Autodesk Inventor part; units mm, degrees
ref_plane "YZ Plane" through (0, 0, 0) normal (1, 0, 0) x (0, 1, 0)
ref_plane "XZ Plane" through (0, 0, 0) normal (0, 1, 0) x (-1, 0, 0)
ref_plane "XY Plane" through (0, 0, 0) normal (0, 0, 1) x (1, 0, 0)
sketch "Sketch1" plane through (0, 0, 0) normal (0, 1, 0) x (-1, 0, 0)
  circle A0 centre (225.7737, 188.8152) radius 1.5
  circle A1 centre (325.7737, 262.422) radius 1.5
  circle A2 centre (374.8449, 262.422) radius 1.5
  circle A3 centre (374.8449, 188.8152) radius 1.5
  circle A4 centre (274.8449, 38.8152) radius 1.5
  circle A5 centre (225.7737, 38.8152) radius 1.5
  circle A6 centre (225.7737, 112.422) radius 1.5
  circle A7 centre (325.7737, 38.8152) radius 1.5
  circle A8 centre (374.8449, 38.8152) radius 1.5
  circle A9 centre (374.8449, 112.422) radius 1.5
  line L0 (200.3093, 45.6186) -> (211.8093, 45.6186)
  line L1 (211.8093, 45.6186) -> (223.3093, 45.6186)
  line L2 (377.3093, 45.6186) -> (388.8093, 45.6186)
  line L3 (388.8093, 45.6186) -> (400.3093, 45.6186)
  line L4 (200.3093, 195.6186) -> (211.8093, 195.6186)
  line L5 (211.8093, 195.6186) -> (223.3093, 195.6186)
  line L6 (377.3093, 195.6186) -> (388.8093, 195.6186)
  line L7 (388.8093, 195.6186) -> (400.3093, 195.6186)
  line L8 (294.3093, 194.1186) -> (306.3093, 194.1186)
  line L9 (306.3093, 194.1186) -> (306.3093, 220.1186)
  line L10 (306.3093, 220.1186) -> (294.3093, 220.1186)
  line L11 (294.3093, 220.1186) -> (294.3093, 194.1186)
  arc A10 (278.5735, 87.7325) -> (322.2559, 87.7325) centre (300.4147, 87.7325) ccw
  circle A11 centre (300.4147, 262.422) radius 10
  line L12 (322.2559, 87.7325) -> (322.2559, 139.8246)
  line L13 (322.2559, 139.8246) -> (278.5735, 139.8246)
  line L14 (278.5735, 139.8246) -> (278.5735, 87.7325)
  circle A12 centre (274.8449, 262.422) radius 1.5
  circle A13 centre (225.7737, 262.422) radius 1.5
  line L15 (238.3093, 105.6186) -> (238.3093, 94.1186)
  line L16 (235.3093, 82.6186) -> (238.3093, 82.6186)
  line L17 (238.3093, 82.6186) -> (238.3093, 94.1186)
  line L18 (362.3093, 105.6186) -> (362.3093, 94.1186)
  line L19 (365.3093, 82.6186) -> (362.3093, 82.6186)
  line L20 (362.3093, 82.6186) -> (362.3093, 94.1186)
  line L21 (235.3093, 195.6186) -> (238.3093, 195.6186)
  line L22 (238.3093, 195.6186) -> (238.3093, 207.1186)
  line L23 (235.3093, 218.6186) -> (238.3093, 218.6186)
  line L24 (238.3093, 218.6186) -> (238.3093, 207.1186)
  line L25 (365.3093, 195.6186) -> (362.3093, 195.6186)
  line L26 (362.3093, 195.6186) -> (362.3093, 207.1186)
  line L27 (365.3093, 218.6186) -> (362.3093, 218.6186)
  line L28 (362.3093, 218.6186) -> (362.3093, 207.1186)
  line L29 (365.3093, 105.6186) -> (362.3093, 105.6186)
  arc A14 (300.3093, 0.6186) -> (400.3093, 38.8152) centre (300.3093, 150.6186) ccw
  arc A15 (200.3093, 38.8152) -> (300.3093, 0.6186) centre (300.3093, 150.6186) ccw
  line L30 (235.3093, 105.6186) -> (200.3093, 105.6186)
  line L31 (200.3093, 45.6186) -> (235.3093, 45.6186)
  line L32 (235.3093, 45.6186) -> (235.3093, 82.6186)
  arc A16 (300.3093, 300.6186) -> (200.3093, 262.422) centre (300.3093, 150.6186) ccw
  line L33 (235.3093, 195.6186) -> (200.3093, 195.6186)
  line L34 (200.3093, 255.6186) -> (235.3093, 255.6186)
  line L35 (235.3093, 255.6186) -> (235.3093, 218.6186)
  line L36 (365.3093, 105.6186) -> (400.3093, 105.6186)
  line L37 (400.3093, 45.6186) -> (365.3093, 45.6186)
  line L38 (365.3093, 45.6186) -> (365.3093, 82.6186)
  arc A17 (400.3093, 262.422) -> (300.3093, 300.6186) centre (300.3093, 150.6186) ccw
  line L39 (365.3093, 195.6186) -> (400.3093, 195.6186)
  line L40 (400.3093, 255.6186) -> (365.3093, 255.6186)
  line L41 (365.3093, 255.6186) -> (365.3093, 218.6186)
  line L42 (235.3093, 105.6186) -> (238.3093, 105.6186)
  line L43 (339.9093, 94.1186) -> (339.9093, 105.6186)
  line L44 (339.9093, 105.6186) -> (342.9093, 105.6186)
  line L45 (342.9093, 105.6186) -> (342.9093, 94.1186)
  line L46 (339.9093, 94.1186) -> (339.9093, 82.6186)
  line L47 (339.9093, 82.6186) -> (342.9093, 82.6186)
  line L48 (342.9093, 82.6186) -> (342.9093, 94.1186)
  line L49 (339.9093, 207.1186) -> (339.9093, 195.6186)
  line L50 (339.9093, 195.6186) -> (342.9093, 195.6186)
  line L51 (342.9093, 195.6186) -> (342.9093, 207.1186)
  line L52 (339.9093, 207.1186) -> (339.9093, 218.6186)
  line L53 (339.9093, 218.6186) -> (342.9093, 218.6186)
  line L54 (342.9093, 218.6186) -> (342.9093, 207.1186)
  line L55 (260.7093, 94.1186) -> (260.7093, 105.6186)
  line L56 (260.7093, 105.6186) -> (257.7093, 105.6186)
  line L57 (257.7093, 105.6186) -> (257.7093, 94.1186)
  line L58 (260.7093, 94.1186) -> (260.7093, 82.6186)
  line L59 (260.7093, 82.6186) -> (257.7093, 82.6186)
  line L60 (257.7093, 82.6186) -> (257.7093, 94.1186)
  line L61 (260.7093, 207.1186) -> (260.7093, 195.6186)
  line L62 (260.7093, 195.6186) -> (257.7093, 195.6186)
  line L63 (257.7093, 195.6186) -> (257.7093, 207.1186)
  line L64 (260.7093, 207.1186) -> (260.7093, 218.6186)
  line L65 (260.7093, 218.6186) -> (257.7093, 218.6186)
  line L66 (257.7093, 218.6186) -> (257.7093, 207.1186)
  line L67 (400.3093, 150.6186) -> (400.3093, 105.6186)
  line L68 (400.3093, 45.6186) -> (400.3093, 38.8152)
  line L69 (211.8093, 0.6186) -> (223.3093, 0.6186)
  line L70 (400.3093, 0.6186) -> (362.3093, 0.6186)
  line L71 (400.3093, 150.6186) -> (400.3093, 195.6186)
  line L72 (400.3093, 255.6186) -> (400.3093, 262.422)
  line L73 (200.3093, 150.6186) -> (200.3093, 195.6186)
  line L74 (200.3093, 150.6186) -> (200.3093, 195.6186)
  line L75 (200.3093, 255.6186) -> (200.3093, 262.422)
  line L76 (200.3093, 255.6186) -> (200.3093, 262.422)
  line L77 (200.3093, 150.6186) -> (200.3093, 105.6186)
  line L78 (200.3093, 45.6186) -> (200.3093, 38.8152)
  line L79 (200.3093, 150.6186) -> (200.3093, 105.6186)
  line L80 (200.3093, 45.6186) -> (200.3093, 38.8152)
extrude "Extrusion1" add sketch "Sketch1" along normal blind 3
properties part number "ChasisSuperior"
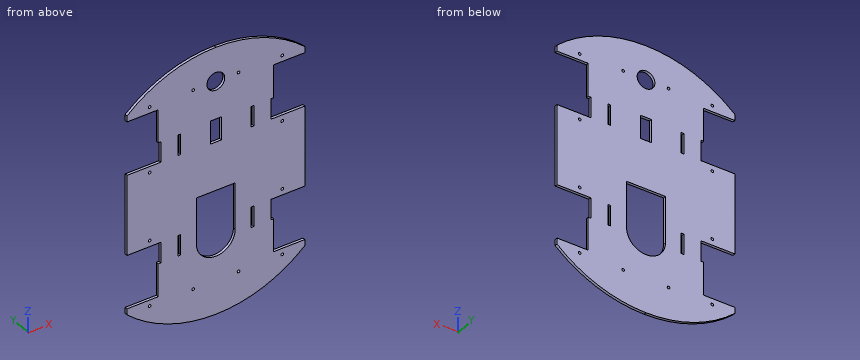
The model under review builds one solid part; all positions refer to its coordinate system, in mm. Coordinates: 2 decimals unless noted, no trailing zeros. Write each loop counter-clockwise with the first axis right and the second up, starting at its lowest first coordinate (ties: lowest second). Pieces come first, ordered by that corner, then holes. Notation, with made-up numbers: (29, -11.5) - (57, -11.5) arc R21 ccw to (57, -5.5) - close; hole circle Ø9 at (-9, 56.25). An arc over 180 degrees is marked (long way). Answer in a Markdown table with one row per item. Add a question column.
Q1. Consider section D-D on y = 1.45. Give the number of separate pieces and of enclosed holes in the cut face, then the cut area to 3 significant figures.
Q2. Consider section B-B on x = -318. Give the boundary of the cut face in (y, z), then the cut area to 3 significant figures.
Q3. Clearance check with flat-ended pins moving along their axes: pin 1 (0.9 mm diameter, centred on y = 1, z = 209.5, fed in from -X); pin 2 (0.9 mm diameter, centred on x = -383, y = 2, fed in from -Z); pin 3 (1.5 mm diameter, centred on x = -236.5, y = 2, fed in from -Z). State where each tip first meets the part, or that it passes through.
Q4. Consider section C-C on z = 228.5. Give the boundary of the cut face in (x, y).
Q5. Consider section A-A on z = 69.5. Give the boundary of the cut face in (x, y).
Q6. To check wall thickness, follow line 1 along X through (y, z) = (1.3, 89.5); line 2 along Z through (x, y) = (-234.5, 1.5); line 3 along X through (y, z) = (0.7, 111.5). State the ranges of each line that lie inside material, in increasing order. Write a range as from..to.
Answers below:
| question | item | result |
|---|---|---|
| 1 | separate pieces | 1 |
| 1 | enclosed holes | 19 |
| 1 | area | 42,500 mm² |
| 2 | outline | (0, 1.67) - (3, 1.67) - (3, 74.78) - (0, 74.78) - close; (0, 139.82) - (3, 139.82) - (3, 299.57) - (0, 299.57) - close |
| 2 | area | 699 mm² |
| 3 | pin 1 | x = -362.31 |
| 3 | pin 2 | z = 25.17 |
| 3 | pin 3 | z = 14.52 |
| 4 | outline | (-365.31, 0) - (-235.31, 0) - (-235.31, 3) - (-365.31, 3) - close |
| 5 | outline | (-365.31, 0) - (-312.44, 0) - (-312.44, 3) - (-365.31, 3) - close; (-288.39, 0) - (-235.31, 0) - (-235.31, 3) - (-288.39, 3) - close |
| 6 | line 1 | -362.31..-342.91, -339.91..-322.26, -278.57..-260.71, -257.71..-238.31 |
| 6 | line 2 | 15.83..45.62, 105.62..195.62, 255.62..285.41 |
| 6 | line 3 | -400.31..-376.03, -373.66..-322.26, -278.57..-226.96, -224.59..-200.31 |
